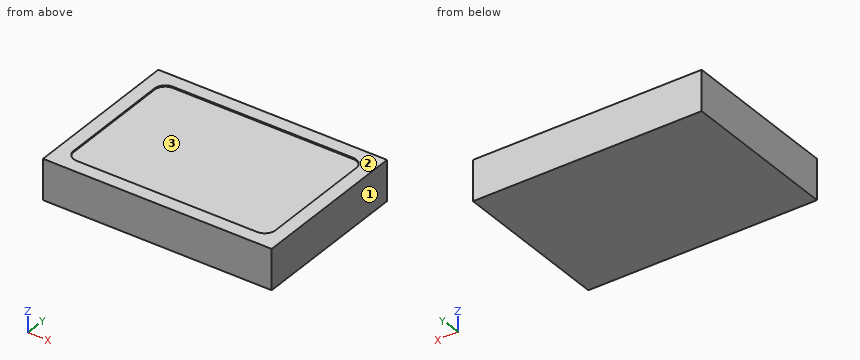
```python
from build123d import *

# Parameters (mm, degrees)
F0_W     = 34
F0_H     = 24
F0_W_2   = 30
F0_H_2   = 20
F1_DEPTH = 6
F2_DEPTH = 0.2
F3_R     = 1.5875


with BuildPart() as f1:
    # F0 (on Top) → F1 (new body)
    with BuildSketch(Plane.XY):
        with Locations((15, -10)):
            Rectangle(F0_W, F0_H)
        with Locations((15, -10)):
            Rectangle(F0_W_2, F0_H_2, mode=Mode.SUBTRACT)
        with Locations((15, -10)):
            Rectangle(F0_W_2, F0_H_2)
    extrude(amount=-F1_DEPTH)

    # F0 (on Top) → F2 (cut)
    with BuildSketch(Plane.XY):
        with Locations((15, -10)):
            Rectangle(F0_W_2, F0_H_2)
    extrude(amount=-F2_DEPTH, mode=Mode.SUBTRACT)

    # F3
    f3_edges = [f1.edges().sort_by_distance(p)[0] for p in [
        (0, 0, -0.1),
        (30, 0, -0.1),
        (30, -20, -0.1),
        (0, -20, -0.1),
    ]]
    fillet(f3_edges, radius=F3_R)


solid = f1.part
```
Could you check a few things on this model? Use its own coordinates, in mm. Face numbers are marked on the shaded views. Coordinates: 2 decimals unless noted, no trailing zeros. Order: outer loops, then holes, each group sorted by start corner. A loop starts at its lowest first (then second) coordinate and runs counter-clockwise, first axis right, second up. Notation, with made-up numbers: M 21.5,39 L 34.5,39 A30 ccw 34.5,63 Z; hole C -32,63.25 d8. An arc over 180 degrees is marked long. Use one line per item in the form item = value. Start each with the question number.
1. Please list where this line runs through material, in increasing order: line 1 (Z direction, x = 25, y = -7).
2. For pin 1 (8 mm diameter, centred on x = 20, y = -7.5, fed in from +Z), with a flat end and sliding along its axis, tell me the tip position at first contact or that it passes through.
3. We'd pull the mould along X, two halves only. Please class the marked faces 1, 2 and 3: +X half, -X half, draft (parallel to the pull), parting line (faces both ways), or undercut.
4. Suppose I cut it at A-A on y = -14.75. Write out the boundary of the cut face in (x, z), then the cut area to 3 significant figures.
5. Suppose I cut it at B-B on x = 16. Write out the boundary of the cut face in (y, z).
Geometry says:
q1.line_1 = -6 to -0.2
q2.pin_1 = -0.2
q3.face_1 = +X half
q3.face_2 = draft
q3.face_3 = undercut
q4.outline = M -2,-6 L 32,-6 L 32,0 L 30,0 L 30,-0.2 L 0,-0.2 L 0,0 L -2,0 Z
q4.area = 198 mm^2
q5.outline = M -22,-6 L 2,-6 L 2,0 L 0,0 L 0,-0.2 L -20,-0.2 L -20,0 L -22,0 Z
